Check sheet for the modelled part. Datum: model origin and axes. Units: mm. A direction names the side the tool comes from. Round coordinates to 2 decimals unless told otherwise and drop trailing zeros. Write each loop counter-clockwise with the first axis right and the second up, starting at its lowest first coordinate (ties: lowest second). Pieces come first, ordered by that corner, then holes. Notation, with made-up numbers: (24, 0) -> (47, 0) arc R15 cw to (47, 8) -> close; hole circle Ø1 at (-13.75, -38.5). An arc over 180 degrees is marked (long way). Use one line per item in the form item = value. Start each with the question number.
```python
from build123d import *

# Parameters (mm, degrees)
F1_DEPTH = 400


# Not quite as in the source:
# - a feature names something its author has since deleted; it is built from what else it names


with BuildPart() as f1:
    # F0 (on Front) → F1 (new body)
    with BuildSketch(Plane.XZ):
        with BuildLine():
            Line((-292.9289321881, -7.0710678119), (-300, 0))
            Line((-300, 0), (-381.3172798365, -81.3172798365))
            ThreePointArc((-381.3172798365, -81.3172798365), (-384.2462120246, -88.3883476483), (-381.3172798365, -95.4594154602))
            Line((-381.3172798365, -95.4594154602), (-155.0431098568, -321.7335854399))
            ThreePointArc((-155.0431098568, -321.7335854399), (-147.9720420449, -324.662517628), (-140.900974233, -321.7335854399))
            Line((-140.900974233, -321.7335854399), (-103.7778682207, -284.6104794276))
            Line((-103.7778682207, -284.6104794276), (-59.5836943966, -240.4163056034))
            Line((-59.5836943966, -240.4163056034), (-66.6547622084, -233.3452377916))
            Line((-66.6547622085, -233.3452377916), (-147.9720420449, -314.662517628))
            Line((-147.9720420449, -314.662517628), (-374.2462120246, -88.3883476483))
            Line((-374.2462120246, -88.3883476483), (-292.9289321882, -7.0710678119))
        make_face()
        with BuildLine():
            Line((-152.9289321881, 147.0710678119), (-300, 0))
            Line((-300, 0), (-292.9289321881, -7.0710678119))
            Line((-292.9289321881, -7.0710678119), (-150, -150))
            Line((-150, -150), (-66.6547622084, -233.3452377916))
            Line((-66.6547622084, -233.3452377916), (-59.5836943966, -240.4163056034))
            Line((-59.5836943966, -240.4163056034), (-7.0710678119, -292.9289321881))
            ThreePointArc((-7.0710678119, -292.9289321881), (0, -295.8578643763), (7.0710678119, -292.9289321881))
            Line((7.0710678119, -292.9289321881), (59.5836943966, -240.4163056034))
            Line((59.5836943966, -240.4163056034), (66.6547622084, -233.3452377916))
            Line((66.6547622084, -233.3452377916), (150, -150))
            Line((150, -150), (225.0000048894, -74.9999951106))
            Line((225.0000048894, -74.9999951106), (292.9289321881, -7.0710678119))
            Line((292.9289321881, -7.0710678119), (300, 0))
            Line((300, 0), (152.9289321881, 147.0710678119))
            ThreePointArc((152.9289321881, 147.0710678119), (149.6846986999, 149.2387953251), (145.8578643763, 150))
            Line((145.8578643763, 150), (-145.8578643763, 150))
            ThreePointArc((-145.8578643763, 150), (-149.6846986999, 149.2387953251), (-152.9289321881, 147.0710678119))
        make_face()
        with BuildLine():
            ThreePointArc((7.0710678119, -278.7867965644), (0, -281.7157287525), (-7.0710678119, -278.7867965644))
            Line((-7.0710678119, -278.7867965644), (-125.8578643763, -160))
            Line((-125.8578643763, -160), (-135.8578643763, -150))
            Line((-135.8578643763, -150), (-210.8578643763, -75))
            Line((-210.8578643763, -75), (-285.8578643763, 0))
            Line((-285.8578643763, 0), (-148.7867965644, 137.0710678118))
            ThreePointArc((-148.7867965644, 137.0710678118), (-145.5425630762, 139.2387953251), (-141.7157287526, 140))
            Line((-141.7157287526, 140), (141.7157287525, 140))
            ThreePointArc((141.7157287525, 140), (145.5425630762, 139.2387953251), (148.7867965644, 137.0710678119))
            Line((148.7867965644, 137.0710678119), (285.8578643762, 0))
            Line((285.8578643762, 0), (210.8578643762, -75))
            Line((210.8578643762, -75), (135.8578643762, -150))
            Line((135.8578643762, -150), (125.8578643762, -160))
            Line((125.8578643762, -160), (7.0710678119, -278.7867965644))
        make_face(mode=Mode.SUBTRACT)
        with BuildLine():
            ThreePointArc((-140.900974233, -321.7335854399), (-147.9720420449, -324.662517628), (-155.0431098568, -321.7335854399))
            Line((-155.0431098568, -321.7335854399), (-7.0710678119, -469.7056274848))
            ThreePointArc((-7.0710678119, -469.7056274848), (0, -472.6345596729), (7.0710678119, -469.7056274848))
            Line((7.0710678119, -469.7056274848), (155.0431098568, -321.7335854399))
            ThreePointArc((155.0431098568, -321.7335854399), (147.9720420449, -324.662517628), (140.900974233, -321.7335854399))
            Line((140.900974233, -321.7335854399), (0, -462.6345596729))
            Line((0, -462.6345596729), (-140.900974233, -321.7335854399))
        make_face()
        with BuildLine():
            Line((381.3172798364, -81.3172798364), (300, 0))
            Line((300, 0), (292.9289321881, -7.0710678119))
            Line((292.9289321881, -7.0710678118), (374.2462120246, -88.3883476483))
            Line((374.2462120246, -88.3883476483), (147.9720420449, -314.662517628))
            Line((147.9720420449, -314.662517628), (66.6547622084, -233.3452377915))
            Line((66.6547622084, -233.3452377916), (59.5836943966, -240.4163056034))
            Line((59.5836943966, -240.4163056034), (140.900974233, -321.7335854399))
            ThreePointArc((140.900974233, -321.7335854399), (147.9720420449, -324.662517628), (155.0431098568, -321.7335854399))
            Line((155.0431098568, -321.7335854399), (381.3172798364, -95.4594154602))
            ThreePointArc((381.3172798364, -95.4594154602), (384.2462120246, -88.3883476483), (381.3172798364, -81.3172798364))
        make_face()
        Polygon((-135.8578643763, -150), (-125.8578643763, -160), (125.8578643762, -160), (135.8578643762, -150), align=None)
    extrude(amount=F1_DEPTH)


solid = f1.part
```
1. Depth check by flat-ended pin: pin 1 (5 mm diameter, centred on x = 220.5, y = -59.5, fed in from +Z); pin 2 (1.5 mm diameter, centred on y = -272.5, z = -36, fed in from +X); pin 3 (8 mm diameter, centred on y = -144.5, z = -173, fed in from +X). Enter the tip coordinate at first touch or a pass-through.
2. Tool access check on faces 1 (the face through (178, -197, -122)), 2 (the face through (191.574, -197.2, -285.202)). Record the directions out of +Z, -Z, +X, -X, +Y, -Y that give a thin tool (end or side, any length) a straight path to the whole face; none if there is none.
3. Sectioned sample at D-D (z = -262). Enter the section's corners in (x, y), and give its area (3 significant figures).
4. Sectioned sample at C-C (x = -167). Enter the section's corners in (y, z).
5. Mould release check, pull along Z, two halves, no side actions. Record for faces 3 (the face through (2, -197, 150)), 4 (the face through (-196.814, -197.2, -279.963)), 5 (the face through (-2, -197, 140)): +Z half, -Z half, draft (parallel to the pull), parting line (faces both ways), or undercut.
6. Sectioned sample at B-B (x = -320.5). Enter the section's corners in (y, z), and give its area (3 significant figures).
7. Scan lines: probe 1 along Z at (x, y) = (-15.5, -318.5); probe 2 along Z at (x, y) = (22, -230); probe 3 along X at (y, z) = (-362, -17). Record each from-to range of solid material in increasing order.
8. Sectioned sample at A-A (z = -29). Enter the section's corners in (x, y).
Returned:
q1.pin_1 = 82
q1.pin_2 = 336.75
q1.pin_3 = 307.78
q2.face_1 = +Y, -Y
q2.face_2 = -Z, +X, +Y, -Y
q3.outline = (-214.78, -400) -> (-200.63, -400) -> (-200.63, 0) -> (-214.78, 0) -> close; (-95.31, -400) -> (-81.17, -400) -> (-81.17, 0) -> (-95.31, 0) -> close; (-38, -400) -> (-23.86, -400) -> (-23.86, 0) -> (-38, 0) -> close; (23.86, -400) -> (38, -400) -> (38, 0) -> (23.86, 0) -> close; (81.17, -400) -> (95.31, -400) -> (95.31, 0) -> (81.17, 0) -> close; (200.63, -400) -> (214.78, -400) -> (214.78, 0) -> (200.63, 0) -> close
q3.area = 33,900 mm^2
q4.outline = (-400, -309.78) -> (0, -309.78) -> (0, -295.63) -> (-400, -295.63) -> close; (-400, -133) -> (0, -133) -> (0, -118.86) -> (-400, -118.86) -> close; (-400, 118.86) -> (0, 118.86) -> (0, 133) -> (-400, 133) -> close
q5.face_3 = +Z half
q5.face_4 = -Z half
q5.face_5 = undercut
q6.outline = (-400, -156.28) -> (0, -156.28) -> (0, -142.13) -> (-400, -142.13) -> close; (-400, -34.64) -> (0, -34.64) -> (0, -20.5) -> (-400, -20.5) -> close
q6.area = 11,300 mm^2
q7.probe_1 = -461.28 to -447.13, -284.5 to -270.36, -160 to -150, 140 to 150
q7.probe_2 = -454.78 to -440.63, -278 to -263.86, -160 to -150, 140 to 150
q7.probe_3 = -317 to -302.86, -283 to -268.86, 268.86 to 283, 302.86 to 317
q8.outline = (-329, -400) -> (-314.86, -400) -> (-314.86, 0) -> (-329, 0) -> close; (-271, -400) -> (-256.86, -400) -> (-256.86, 0) -> (-271, 0) -> close; (256.86, -400) -> (271, -400) -> (271, 0) -> (256.86, 0) -> close; (314.86, -400) -> (329, -400) -> (329, 0) -> (314.86, 0) -> close
